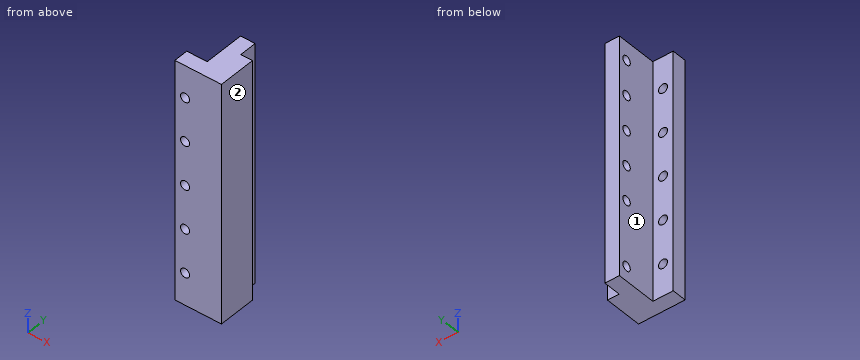
from build123d import *

# Parameters (mm, degrees)
EXTRUDE_1_DEPTH        = 82
SKETCH_2_R             = 1.55
CUT_EXTRUDE_1_DEPTH    = 84.886828525
SKETCH_3_R             = 1.55
CUT_EXTRUDE_2_DEPTH    = 85.711274338
PATTERN_LINEAR_1_COUNT = 5
PATTERN_LINEAR_1_PITCH = 15


with BuildPart() as part:
    # 草圖1 → 填料-伸長1 (new body)
    with BuildSketch(Plane.XY):
        Polygon((-9, 6), (-9, -8), (-16, -8), (-16, -13), (0, -13), (0, 0), (-4, 0), (-4, 6), align=None)
    extrude(amount=EXTRUDE_1_DEPTH)

    # 草圖2 → 除料-伸長1 (cut, through all)
    with BuildSketch(Plane(origin=(-4, 0, 0), x_dir=(0, 0, -1), z_dir=(1, 0, 0))):
        with Locations((-75.5, 3)):
            Circle(SKETCH_2_R)
        with Locations((-63.5, 3)):
            Circle(SKETCH_2_R)
        with Locations((-51.5, 3)):
            Circle(SKETCH_2_R)
        with Locations((-39.5, 3)):
            Circle(SKETCH_2_R)
        with Locations((-27.5, 3)):
            Circle(SKETCH_2_R)
        with Locations((-5, 3)):
            Circle(SKETCH_2_R)
    extrude(amount=-CUT_EXTRUDE_1_DEPTH, mode=Mode.SUBTRACT)

    # 草圖3 → 除料-伸長2 (cut, through all)
    with BuildSketch(Plane(origin=(0, -8, 0), x_dir=(1, 0, 0), z_dir=(0, 1, 0))):
        with Locations(Location((-12.5, -11, 0), (0, 0, 180))):
            Circle(SKETCH_3_R)
    cut_extrude_2 = extrude(amount=-CUT_EXTRUDE_2_DEPTH, mode=Mode.SUBTRACT)

    # 直線複製排列1: 除料-伸長2 ×5
    with Locations(*[(0, 0, i * PATTERN_LINEAR_1_PITCH) for i in range(1, PATTERN_LINEAR_1_COUNT)]):
        add(cut_extrude_2, mode=Mode.SUBTRACT)


solid = part.part
Build history of the part. All positions in model axes, mm. Face numbers are marked on the shaded views. A direction names the side the tool comes from. Round coordinates to 2 decimals unless told otherwise and drop trailing zeros. Loops run counter-clockwise (first coordinate to the right, second up) from the corner with the lowest first, then second, coordinate; pieces in that order, holes last. Notation, with made-up numbers: (59.25, -31.5) -> (96.25, -31.5) arc R22 cw to (96.25, -22.5) -> close; hole circle Ø10 at (-30.5, -32.75). An arc over 180 degrees is marked (long way). Use CSV: the item, a comma, the result in double quotes. Start each with the question number.
Q1. Drill centre lines: L1, parallel to Z at x = -12.5, y = -11.8; L2, parallel to Y at x = -7.75, z = 63.5; L3, parallel to X at y = -11.25, z = 71. Where is each one in solid material? Low to high.
Q2. Saw through at B-B on y = 3. Give the cut face in (x, z).
Q3. Saw through at C-C on x = -7. Give the cut face in (y, z), and give its area (3 significant figures).
Q4. Flat gauge pins, fed straight in: pin 1 Ø5 at (y, z) = (1.5, 29) entering from +X; pin 2 Ø7 at (y, z) = (-2, 24) entering from -X; pin 3 Ø5 at (y, z) = (3, 39.5) entering from +X; pin 4 Ø3.5 at (x, z) = (-12.5, 41) entering from +Y. Where does each tip first touch, or does it go through?
Q5. Saw through at A-A on z = 11. Give the cut face in (x, y), and give its area (4 significant figures).
Q6. Saw through at D-D on y = -9.75. Give the cut face in (x, z).
Q7. Which spindle directions (+Z, -Z, +X, -X, +Y, -Y) get a long thin tool onto all of the face, cutting with end or side? Do the marked faces 1 and 2. Say none if no direction does.
Solutions:
1,L1,"z = 0 to 9.45, 12.55 to 24.45, 27.55 to 39.45, 42.55 to 54.45, 57.55 to 69.45, 72.55 to 82"
1,L2,"y = -13 to 1.45, 4.55 to 6"
1,L3,"x = -16 to -14.05, -10.95 to 0"
2,outline,"(-9, 0) -> (-4, 0) -> (-4, 3.45) -> (-9, 3.45) -> close; (-9, 6.55) -> (-4, 6.55) -> (-4, 25.95) -> (-9, 25.95) -> close; (-9, 29.05) -> (-4, 29.05) -> (-4, 37.95) -> (-9, 37.95) -> close; (-9, 41.05) -> (-4, 41.05) -> (-4, 49.95) -> (-9, 49.95) -> close; (-9, 53.05) -> (-4, 53.05) -> (-4, 61.95) -> (-9, 61.95) -> close; (-9, 65.05) -> (-4, 65.05) -> (-4, 73.95) -> (-9, 73.95) -> close; (-9, 77.05) -> (-4, 77.05) -> (-4, 82) -> (-9, 82) -> close"
3,outline,"(-13, 0) -> (6, 0) -> (6, 82) -> (-13, 82) -> close; hole circle Ø3.1 at (3, 5); hole circle Ø3.1 at (3, 27.5); hole circle Ø3.1 at (3, 39.5); hole circle Ø3.1 at (3, 51.5); hole circle Ø3.1 at (3, 63.5); hole circle Ø3.1 at (3, 75.5)"
3,area,"1,510 mm^2"
4,pin 1,"stops at x = 0"
4,pin 2,"stops at x = -9"
4,pin 3,"stops at x = -4"
4,pin 4,"stops at y = -8"
5,outline,"(-16, -13) -> (-14.05, -13) -> (-14.05, -8) -> (-16, -8) -> close; (-10.95, -13) -> (0, -13) -> (0, 0) -> (-4, 0) -> (-4, 6) -> (-9, 6) -> (-9, -8) -> (-10.95, -8) -> close"
5,area,"166.5 mm^2"
6,outline,"(-16, 0) -> (0, 0) -> (0, 82) -> (-16, 82) -> close; hole circle Ø3.1 at (-12.5, 11); hole circle Ø3.1 at (-12.5, 26); hole circle Ø3.1 at (-12.5, 41); hole circle Ø3.1 at (-12.5, 56); hole circle Ø3.1 at (-12.5, 71)"
7,face 1,"+Z, -Z, -X, +Y"
7,face 2,"+Z, -Z, +X, +Y, -Y"
